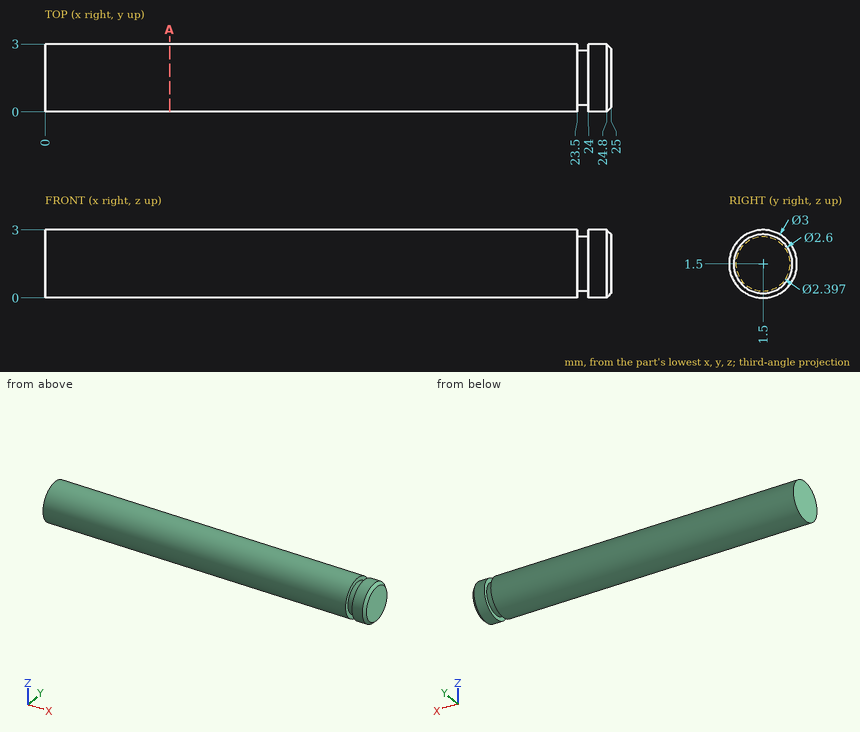
For this review, use the dimensioned drawing (mm, ordinates from the lowest corner) and the shaded views. Round coordinates to 2 decimals unless told otherwise and drop trailing zeros. Write each loop counter-clockwise with the first axis right and the second up, starting at its lowest first coordinate (ties: lowest second). Pieces come first, ordered by that corner, then holes. Notation, with made-up numbers: (9, 34.5) -> (25, 34.5) arc R20 ccw to (25, 41.5) -> close; hole circle Ø8 at (22.25, 37). An arc over 180 degrees is marked (long way). Use CSV: the item, a comma, the result in double quotes.
(1) To check wall thickness, follow L1, parallel to X at y = 0.95, z = 2.6; L2, parallel to Y at x = 2.75, z = 1.4; L3, parallel to Z at x = 15.75, y = 1.9 (1 decimal). State the ranges of each line that lie inside material, in increasing order. Write a range as [from, to].
Computed values:
L1,"[0, 23.5], [24, 25]"
L2,"[0, 3]"
L3,"[0.1, 2.9]"
(2) Clearance check with flat-ended pins moving along their axes: P1, Ø1.5, axis at y = 2, z = 1.5, coming from the -X side; P2, Ø1.5, axis at x = 6.5, z = 0.5, coming from the +Y side. State where each tip first meets the part, or that it passes through.
Computed values:
P1,"x = 0"
P2,"y = 2.98"
(3) Consider section A-A, the plane x = 5.5. Give the boundary of the cut face in (y, z).
Computed values:
outline,"circle Ø3 at (1.5, 1.5)"
